Read the model definition and answer for the solid it produces. Units are mm, in the model's axes. Face numbers are marked on the shaded views. A direction names the side the tool comes from. Round coordinates to 2 decimals unless told otherwise and drop trailing zeros. Write each loop counter-clockwise with the first axis right and the second up, starting at its lowest first coordinate (ties: lowest second). Pieces come first, ordered by that corner, then holes. Notation, with made-up numbers: (-34, -13) -> (6, -13) arc R16 ccw to (6, 5) -> close; hole circle Ø5 at (-12.75, 16). An arc over 180 degrees is marked (long way). Return JSON: item names as keys, results as strings. Group by question number.
(1) Straight lines are drawn through the part: line 1 (Z direction, x = 10.5, y = 43.5); line 2 (Y direction, x = 7.5, z = 29.75); line 3 (Z direction, x = 7.25, y = 10). For each, find the intervals that lie inside material, in ascending order.
(2) A cutting plane is placed at C-C on y = -22. Give the vertices of the cut face in (x, z).
(3) A cutting plane is placed at D-D on z = 24. Give the vertices of the cut face in (x, y), then the cut area to 3 significant figures.
(4) A cutting plane is placed at B-B on z = 11. Give the vertices of the cut face in (x, y), then the cut area to 3 significant figures.
(5) For the marked faces 1 and 2, determine the directions among +Z, -Z, +X, -X, +Y, -Y from which every point of the face is accessible in a straight line to the end or side of a thin tool.
(6) Given pin 1 (3 mm diameter, centred on x = 7.5, y = 0, fed in from +Z); pin 2 (1 mm diameter, centred on x = 8, z = 20, fed in from -Y); pin 3 (8 mm diameter, centred on x = 20, y = -27, fed in from +Z), each flat-ended and moving along its own axis, determine where each tip first touches the part or whether it passes through.
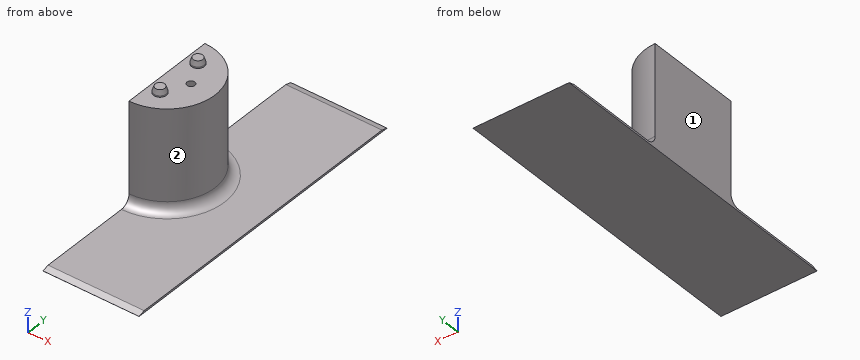
```python
from build123d import *

# Parameters (mm, degrees)
SKETCH001_W        = 30
SKETCH001_H        = 98
PAD001_DEPTH       = 0.6
CHAMFER_1_SIZE2    = 2
CHAMFER_1_SIZE     = 0.59
CHAMFER_2_SIZE2    = 2
CHAMFER_2_SIZE     = 0.59
PAD002_DEPTH       = 32
FILLET_R           = 3
SKETCH003_R        = 1.2
HOLE_DEPTH         = 12
HOLE_TIPS_R        = 1.2
SKETCH004_R        = 1.99
PAD003_DEPTH       = 1.95
CHAMFER001_1_SIZE2 = 0.5
CHAMFER001_1_SIZE  = 1.5
CHAMFER001_2_SIZE2 = 0.5
CHAMFER001_2_SIZE  = 1.5


with BuildPart() as part:
    # Sketch001 → Pad001 (new body)
    with BuildSketch(Plane.XY):
        with Locations((15, 0)):
            Rectangle(SKETCH001_W, SKETCH001_H)
    extrude(amount=PAD001_DEPTH)

    # Chamfer 1
    chamfer_1_edges = [part.edges().sort_by_distance(p)[0] for p in [
        (15, -49, 0.6),
    ]]
    chamfer_1_side = part.faces().sort_by_distance((15, -49, 0.3))[0]
    chamfer(chamfer_1_edges, length=CHAMFER_1_SIZE, length2=CHAMFER_1_SIZE2, reference=chamfer_1_side)

    # Chamfer 2
    chamfer_2_edges = [part.edges().sort_by_distance(p)[0] for p in [
        (15, 49, 0.6),
    ]]
    chamfer_2_side = part.faces().sort_by_distance((15, 49, 0.3))[0]
    chamfer(chamfer_2_edges, length=CHAMFER_2_SIZE, length2=CHAMFER_2_SIZE2, reference=chamfer_2_side)

    # Sketch002 → Pad002 (join)
    with BuildSketch(Plane.XY):
        with BuildLine():
            Line((0, -15), (0, 15))
            ThreePointArc((0, -15), (15, 0), (0, 15))
        make_face()
    extrude(amount=PAD002_DEPTH)

    # Fillet
    fillet_edges = [part.edges().sort_by_distance(p)[0] for p in [
        (15, 0, 0.6),
    ]]
    fillet(fillet_edges, radius=FILLET_R)

    # Sketch003 (on Face9 of Fillet) → Hole (cut)
    with BuildSketch(Plane.XY.offset(32)):
        with Locations((7.5, 0)):
            Circle(SKETCH003_R)
    extrude(amount=-HOLE_DEPTH, mode=Mode.SUBTRACT)

    # Hole tips → Hole tip 1 section 0
    with BuildSketch(Plane.XY.offset(20), mode=Mode.PRIVATE) as hole_tip_1_s0:
        with Locations((7.5, 0)):
            Circle(HOLE_TIPS_R)
    loft([hole_tip_1_s0.sketch, Vertex(7.5, 0, 19.278967)], mode=Mode.SUBTRACT)

    # Sketch004 (on Face9 of Hole) → Pad003 (join)
    with BuildSketch(Plane.XY.offset(32)):
        with Locations((3.75, 7.5)):
            Circle(SKETCH004_R)
        with Locations((3.75, -7.5)):
            Circle(SKETCH004_R)
    extrude(amount=PAD003_DEPTH)

    # Chamfer001 1
    chamfer001_1_edges = [part.edges().sort_by_distance(p)[0] for p in [
        (1.76, -7.5, 33.95),
    ]]
    chamfer001_1_side = part.faces().sort_by_distance((1.76, -7.5, 32.975))[0]
    chamfer(chamfer001_1_edges, length=CHAMFER001_1_SIZE, length2=CHAMFER001_1_SIZE2, reference=chamfer001_1_side)

    # Chamfer001 2
    chamfer001_2_edges = [part.edges().sort_by_distance(p)[0] for p in [
        (1.76, 7.5, 33.95),
    ]]
    chamfer001_2_side = part.faces().sort_by_distance((1.76, 7.5, 32.975))[0]
    chamfer(chamfer001_2_edges, length=CHAMFER001_2_SIZE, length2=CHAMFER001_2_SIZE2, reference=chamfer001_2_side)


solid = part.part
```
Checks:
{
 "1": {"line 1": "z = 0 to 0.6", "line 2": "y = -12.99 to -1.2, 1.2 to 12.99", "line 3": "z = 0 to 32"},
 "2": {"outline": "(0, 0) -> (30, 0) -> (30, 0.6) -> (0, 0.6) -> close"},
 "3": {"outline": "(0, -15) arc R15 ccw to (0, 15) -> close; hole circle Ø2.4 at (7.5, 0)", "area": "349 mm^2"},
 "4": {"outline": "(0, -15) arc R15 ccw to (0, 15) -> close", "area": "353 mm^2"},
 "5": {"face 1": "+Z, -Z, -X, +Y, -Y", "face 2": "+Z, +X"},
 "6": {"pin 1": "stops at z = 32", "pin 2": "stops at y = -12.99", "pin 3": "stops at z = 0.6"}
}
